Can you work these out from the model? Positions are in its coordinate system, mm. A direction names the side the tool comes from. Round coordinates to 2 decimals unless told otherwise and drop trailing zeros. Write each loop counter-clockwise with the first axis right and the second up, starting at its lowest first coordinate (ties: lowest second). Pieces come first, ordered by that corner, then holes. Notation, with made-up numbers: M 57,25.25 L 109,25.25 A18 ccw 109,46.25 Z; hole C 7.25,27 d7. An arc over 180 degrees is marked long. Answer in a Markdown table with one row per item. Add a question column.
(1) I'm going to push flat-ended pins straight in: pin 1 (7 mm diameter, centred on x = 0, z = 48.87, fed in from +Y); pin 2 (11.5 mm diameter, centred on x = -1.5, z = -23.5, fed in from -Y); pin 3 (12 mm diameter, centred on y = -27, z = 31, fed in from -X); pin 4 (8 mm diameter, centred on x = 1, y = -10.5, fed in from -Z). Where does each tip first touch, or does it pass through?
(2) Suppose I cut it at D-D, the plane y = -26. Write out the boundary of the cut face in (x, z).
(3) If I drill on probe 1 along Z at (x, y) = (0, -3.3); probe 2 along Z at (x, y) = (-1.5, -4.5); probe 3 along Y at (x, z) = (6, -5.5), over which ranges is the centre line in solid material (lowest first)?
(4) Suppose I cut it at A-A, the plane x = 0. Write out the boundary of the cut face in (y, z).
(5) If we mould it in two halves opening along X, with no side actions, what happens to faces 1 (the face through (0, -45, 29)), 2 (the face through (19, -3, -1)), 3 (the face through (-0.867, -3.042, 44.965))? For each: released by +X, released by -X, zero draft, split by the parting line, or undercut.
(6) Suppose I cut it at B-B, the plane z = 34. Write out the boundary of the cut face in (x, y).
(7) For faces 4 (the face through (0, 0, 1)), 5 (the face through (4.301, -25.227, 35.615)), which set-ups out of +Z, -Z, +X, -X, +Y, -Y let a thin tool reach every point of the face, with its end or its side?
(8) Suppose I cut it at C-C, the plane x = -13.5. Write out the boundary of the cut face in (y, z), then the cut area to 3 significant figures.
from build123d import *

# Parameters (mm, degrees)
F0_W     = 37.999924
F0_H     = 115.010692
F0_R     = 7.99973
F1_DEPTH = 6
F2_DEPTH = 45
F3_R     = 4
F4_DEPTH = 6.001


with BuildPart() as f1:
    # F0 (on Front) → F1 (new body)
    with BuildSketch(Plane.XZ):
        Rectangle(F0_W, F0_H)
        with Locations((0, 28.869588)):
            Circle(F0_R, mode=Mode.SUBTRACT)
    extrude(amount=F1_DEPTH)

    # F0 (on Front) → F2 (join)
    with BuildSketch(Plane.XZ):
        with Locations((0, 28.869588)):
            Circle(F0_R)
    extrude(amount=F2_DEPTH)

    # F3 (on face) → F4 (cut, through all)
    with BuildSketch(Plane.XZ.offset(6)):
        with Locations((0, 48.869588)):
            Circle(F3_R)
        with Locations((0, -28.130412)):
            Circle(F3_R)
    extrude(amount=-F4_DEPTH, mode=Mode.SUBTRACT)


solid = f1.part
Calculated:
| question | item | result |
|---|---|---|
| 1 | pin 1 | through |
| 1 | pin 2 | y = -6 |
| 1 | pin 3 | x = -8 |
| 1 | pin 4 | z = 20.87 |
| 2 | outline | C 0,28.87 d16 |
| 3 | probe 1 | -57.51 to -32.13, -24.13 to 44.87, 52.87 to 57.51 |
| 3 | probe 2 | -57.51 to -31.84, -24.42 to 45.16, 52.58 to 57.51 |
| 3 | probe 3 | -6 to 0 |
| 4 | outline | M -45,20.87 L -6,20.87 L -6,-24.13 L 0,-24.13 L 0,44.87 L -6,44.87 L -6,36.87 L -45,36.87 Z; M -6,-57.51 L 0,-57.51 L 0,-32.13 L -6,-32.13 Z; M -6,52.87 L 0,52.87 L 0,57.51 L -6,57.51 Z |
| 5 | face 1 | zero draft |
| 5 | face 2 | released by +X |
| 5 | face 3 | undercut |
| 6 | outline | M -19,-6 L -6.14,-6 L -6.14,-45 L 6.14,-45 L 6.14,-6 L 19,-6 L 19,0 L -19,0 Z |
| 7 | face 4 | +Z, -Z, +X, -X, +Y |
| 7 | face 5 | -Y |
| 8 | outline | M -6,-57.51 L 0,-57.51 L 0,57.51 L -6,57.51 Z |
| 8 | area | 690 mm² |
